```python
from build123d import *

# Parameters (mm, degrees)
BOSS_EXTRUDE1_DEPTH   = 16.4
F_4_40_TAPPED_HOLE1_D = 2.2606
F_3_0MM_DOWEL_HOLE1_D = 3
F_4_CLEARANCE_HOLE1_D = 3.2639
FILLET1_R             = 2.5
FILLET2_R             = 2


with BuildPart() as part:
    # Sketch1 → Boss-Extrude1 (new body)
    with BuildSketch(Plane(origin=(0, 0, 0), x_dir=(1, 0, 0), z_dir=(0, 1, 0))):
        Polygon((-4, -3), (-4, -20), (4, -20), (4, 20), (-4, 20), (-4, 3), (-44, 3), (-44, -3), align=None)
    extrude(amount=BOSS_EXTRUDE1_DEPTH)

    # #4-40 Tapped Hole1 (through all)
    with Locations(Plane(origin=(0, 16.4, 0), x_dir=(1, 0, 0), z_dir=(0, 1, 0))):
        with Locations((0, 15), (0, -15)):
            Hole(F_4_40_TAPPED_HOLE1_D / 2)

    # Ø3.0mm Dowel Hole1 (through all)
    with Locations(Plane.XY.offset(3)):
        with Locations((-25.91, 8.2)):
            Hole(F_3_0MM_DOWEL_HOLE1_D / 2)

    # #4 Clearance Hole1 (through all)
    with Locations(Plane.XY.offset(3)):
        with Locations((-39, 8.2), (-12.82, 8.2)):
            Hole(F_4_CLEARANCE_HOLE1_D / 2)

    # Fillet1
    fillet1_edges = [part.edges().sort_by_distance(p)[0] for p in [
        (-4, 8.2, 3),
        (-4, 8.2, -3),
    ]]
    fillet(fillet1_edges, radius=FILLET1_R)

    # Fillet2
    fillet2_edges = [part.edges().sort_by_distance(p)[0] for p in [
        (4, 8.2, 20),
        (-4, 8.2, 20),
        (-44, 8.2, 3),
        (-44, 8.2, -3),
        (-4, 8.2, -20),
        (4, 8.2, -20),
    ]]
    fillet(fillet2_edges, radius=FILLET2_R)


solid = part.part
```
Can you work these out from the model? Positions are in its coordinate system, mm. A direction names the side the tool comes from. Round coordinates to 2 decimals unless told otherwise and drop trailing zeros. Loops run counter-clockwise (first coordinate to the right, second up) from the corner with the lowest first, then second, coordinate; pieces in that order, holes last. Notation, with made-up numbers: M 32,18 L 62,18 A12 ccw 62,41 Z; hole C 37,-35.5 d1. An arc over 180 degrees is marked long. Write item = value, one per line. Start each with the question number.
(1) Suppose I cut it at A-A on y = 8.75. Give the number of separate pieces and of enclosed holes in the cut face, plus the area to 3 significant figures.
(2) Suppose I cut it at B-B on z = 15. Write out the boundary of the cut face in (x, y), plus the area to 3 significant figures.
(3) Which directions (+Z, -Z, +X, -X, +Y, -Y) give clear straight access to the entire face, cutting with the end or side of a thin tool? Please do faces 4 (the face through (-24, 6, 3)), 5 (the face through (-4, 8, -12)), 6 (the face through (3.4, 8.31, 19.43)).
(4) Suppose I cut it at C-C on x = -25.91. Write out the boundary of the cut face in (y, z).
(5) Suppose I cut it at D-D on z = 0. Write out the boundary of the cut face in (x, y), plus the area to 3 significant figures.
(6) I'm going to push flat-ended pins straight in: P1, Ø4, axis at x = -21.5, y = 4.5, coming from the +Z side; P2, Ø4, axis at x = -39, y = 8.2, coming from the -Z side; P3, Ø1, axis at x = -34.5, z = -4.5, coming from the +Y side (3 decimals); P4, Ø6, axis at y = 8, z = -9, coming from the -X side. Where does each tip first touch, or does it pass through?
(7) If we mould it in two halves opening along Z, with no side actions, what happens to faces 1 (the face through (-11, 16.4, -2)), 2 (the face through (-0.522, 8.085, 16.003)), 3 (the face through (-4.752, 8.315, -3.713))? For each: released by +Z, released by -Z, zero draft, split by the parting line, or undercut.
(8) I need wall thicknesses on line 1 along Z through (x, y) = (0, 6.75); line 2 along Y through (x, z) = (-25.91, 0.3); line 3 along Y through (x, z) = (-39, -1.5). Which ranges of each line are inside material? Lowest first, please.
Answer block:
q1.separate_pieces = 4
q1.enclosed_holes = 2
q1.area = 496 mm²
q2.outline = M -4,0 L -1.13,0 L -1.13,16.4 L -4,16.4 Z; M 1.13,0 L 4,0 L 4,16.4 L 1.13,16.4 Z
q2.area = 94.1 mm²
q3.face_4 = +Z, -X, +Y, -Y
q3.face_5 = -Z, -X, +Y, -Y
q3.face_6 = +Z, +X, +Y, -Y
q4.outline = M 0,-3 L 6.7,-3 L 6.7,3 L 0,3 Z; M 9.7,-3 L 16.4,-3 L 16.4,3 L 9.7,3 Z
q5.outline = M -44,0 L 4,0 L 4,16.4 L -44,16.4 Z; hole C -39,8.2 d3.26; hole C -25.91,8.2 d3; hole C -12.82,8.2 d3.26
q5.area = 763 mm²
q6.P1 = 3
q6.P2 = -3
q6.P3 = through
q6.P4 = -4
q7.face_1 = zero draft
q7.face_2 = undercut
q7.face_3 = released by -Z
q8.line_1 = -20 to -16.13, -13.87 to 13.87, 16.13 to 20
q8.line_2 = 0 to 6.7, 9.7 to 16.4
q8.line_3 = 0 to 6.57, 9.83 to 16.4
